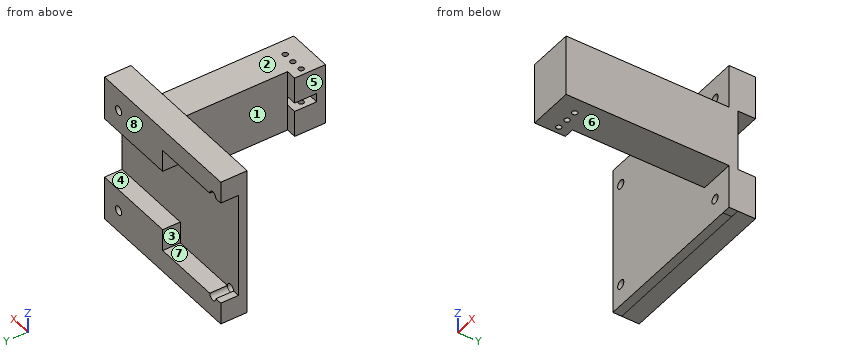
```python
from build123d import *
from build123d.topology import SkipClean

# Parameters (mm, degrees)
SKETCH3_W                = 4.167944103
SKETCH3_H                = 2.5
SKETCH3_R                = 0.3
BOSS_EXTRUDE1_DEPTH      = 3
BOSS_EXTRUDE3_DEPTH      = 3
BOSS_EXTRUDE4_DEPTH      = 8
SKETCH7_R                = 0.5
CUT_EXTRUDE1_DEPTH       = 1
BOSS_EXTRUDE5_DEPTH      = 1
BOSS_EXTRUDE5_DEPTH_BACK = 1
SKETCH8_W                = 4.167944103
SKETCH8_H                = 1
SKETCH8_W_2              = 1
BOSS_EXTRUDE6_START      = -3.5
BOSS_EXTRUDE6_OUTLINE_W  = 4.167944103
BOSS_EXTRUDE6_OUTLINE_H  = 1
BOSS_EXTRUDE6_DEPTH      = 7
BOSS_EXTRUDE7_START      = -3.5
BOSS_EXTRUDE7_OUTLINE_W  = 1
BOSS_EXTRUDE7_OUTLINE_H  = 18.5
BOSS_EXTRUDE7_DEPTH      = 7
BOSS_EXTRUDE8_START      = 2
SKETCH9_R                = 0.5
BOSS_EXTRUDE8_DEPTH      = 2
BOSS_EXTRUDE9_DEPTH      = 8.5
BOSS_EXTRUDE9_DEPTH_BACK = 8.5
SKETCH8_7_W              = 1
SKETCH8_7_H              = 1


# Read off the part's stored shape, not the designer's step: Boss-Extrude6, Boss-Extrude7
with BuildPart() as part:
    # Sketch3 → Boss-Extrude1 (new body)
    with BuildSketch(Plane.XY):
        with Locations((0.002500359, -0.178234892)):
            Rectangle(SKETCH3_W, SKETCH3_H)
        with Locations((-1.297499642, -0.208485146)):
            Circle(SKETCH3_R, mode=Mode.SUBTRACT)
        with Locations((0.002500358, -0.178234892)):
            Circle(SKETCH3_R, mode=Mode.SUBTRACT)
        with Locations((1.302500358, -0.208485146)):
            Circle(SKETCH3_R, mode=Mode.SUBTRACT)
    extrude(amount=BOSS_EXTRUDE1_DEPTH)

    # Sketch6 → Boss-Extrude3 (add)
    with BuildSketch(Plane.XY):
        Polygon((-0.91352759, 1.071765108), (2.08647241, 1.071765108), (2.08647241, 17.071765108), (-15.91352759, 17.071765108), (-15.91352759, 16.071765108), (-0.91352759, 16.071765108), align=None)
    extrude(amount=BOSS_EXTRUDE3_DEPTH)

    # Sketch6_5 → Boss-Extrude4 (add)
    with BuildSketch(Plane.XY):
        Polygon((-0.91352759, 16.071765108), (2.08647241, 16.071765108), (2.08647241, 17.071765108), (-15.91352759, 17.071765108), (-15.91352759, 16.071765108), align=None)
    extrude(amount=BOSS_EXTRUDE4_DEPTH)


with BuildPart() as body_2:
    # Mirror4: mirrored copy
    add(part.part.mirror(Plane(origin=(0, 0, -0.5), x_dir=(1, 0, 0), z_dir=(0, 0, -1))))


with BuildPart() as cut_extrude1_tool:
    # Sketch7 → Cut-Extrude1 (new body)
    with BuildSketch(Plane(origin=(0, 17.071765108, 0), x_dir=(1, 0, 0), z_dir=(0, 1, 0))):
        with Locations(Location((-14.61352759, -5.5, 0), (0, 0, 270))):
            Circle(SKETCH7_R)
        with Locations(Location((-14.61352759, 6.5, 0), (0, 0, 270))):
            Circle(SKETCH7_R)
        with Locations(Location((0.78647241, -5.5, 0), (0, 0, 270))):
            Circle(SKETCH7_R)
        with Locations(Location((0.78647241, 6.5, 0), (0, 0, 270))):
            Circle(SKETCH7_R)
    extrude(amount=-CUT_EXTRUDE1_DEPTH)


with BuildPart() as part_1:
    add(part.part)

    # Cut-Extrude1: cut by cut_extrude1_tool
    add(cut_extrude1_tool.part, mode=Mode.SUBTRACT)



with BuildPart() as body_2_1:
    add(body_2.part)

    # Cut-Extrude1: cut by cut_extrude1_tool
    add(cut_extrude1_tool.part, mode=Mode.SUBTRACT)


with BuildPart() as part_2:
    add(part_1.part)

    add(body_2_1.part)  # Boss-Extrude5 merges body 2
    # Sketch8 → Boss-Extrude5 (add, two sides: drawn at the far end of the back side and taken through both)
    with BuildSketch(Plane(origin=(0, 0, -0.5), x_dir=(-1, 0, 0), z_dir=(0, 0, -1)).offset(-BOSS_EXTRUDE5_DEPTH_BACK)):
        Polygon((-2.08647241, 16.071765108), (-2.08647241, 1.071765108), (0.91352759, 1.071765108), (0.91352759, 16.071765108), (15.91352759, 16.071765108), (15.91352759, 17.071765108), (-2.08647241, 17.071765108), align=None)
        Polygon((-2.08647241, 17.071765108), (-2.08647241, -1.428234892), (-2.08647241, -2.428234892), (-3.08647241, -2.428234892), (-3.08647241, 17.071765108), align=None)
        with Locations((-0.002500359, -1.928234892)):
            Rectangle(SKETCH8_W, SKETCH8_H)
        with Locations((-2.58647241, 16.571765108)):
            Rectangle(SKETCH8_W_2, SKETCH8_H)
    extrude(amount=BOSS_EXTRUDE5_DEPTH + BOSS_EXTRUDE5_DEPTH_BACK)

    # Boss-Extrude6 outline → Boss-Extrude6 (add)
    with BuildSketch(Plane(origin=(0, 0, -0.5), x_dir=(-1, 0, 0), z_dir=(0, 0, -1)).offset(BOSS_EXTRUDE6_START)):
        with Locations((-0.002500359, -1.928234892)):
            Rectangle(BOSS_EXTRUDE6_OUTLINE_W, BOSS_EXTRUDE6_OUTLINE_H)
    extrude(amount=BOSS_EXTRUDE6_DEPTH)

    # Boss-Extrude7 outline → Boss-Extrude7 (add)
    with BuildSketch(Plane(origin=(0, 0, -0.5), x_dir=(-1, 0, 0), z_dir=(0, 0, -1)).offset(BOSS_EXTRUDE7_START)):
        with Locations((-2.58647241, 6.821765108)):
            Rectangle(BOSS_EXTRUDE7_OUTLINE_W, BOSS_EXTRUDE7_OUTLINE_H)
    extrude(amount=BOSS_EXTRUDE7_DEPTH)

    # Sketch9 → Boss-Extrude8 (add)
    # profile 1 of 2: a face of its own
    with SkipClean():  # the faces are left unmerged after this step: merging them gives an invalid solid
        with BuildSketch(Plane(origin=(0, 17.071765108, 0), x_dir=(1, 0, 0), z_dir=(0, 1, 0)).offset(BOSS_EXTRUDE8_START)):
            with BuildLine():
                Line((-6.41352759, 6.5), (-6.41352759, 4))
                Line((-6.41352759, 4), (3.08647241, 4))
                Line((3.08647241, 4), (3.08647241, 9))
                Line((3.08647241, 9), (-15.91352759, 9))
                Line((-15.91352759, 9), (-15.91352759, 6.5))
                Line((-15.91352759, 6.5), (-15.11352759, 6.5))
                ThreePointArc((-15.11352759, 6.5), (-14.61352759, 7), (-14.11352759, 6.5))
                Line((-14.11352759, 6.5), (-6.41352759, 6.5))
            make_face()
            with Locations((0.78647241, 6.5)):
                Circle(SKETCH9_R, mode=Mode.SUBTRACT)
        # profile 2 of 2: a face of its own
        with BuildSketch(Plane(origin=(0, 17.071765108, 0), x_dir=(1, 0, 0), z_dir=(0, 1, 0)).offset(BOSS_EXTRUDE8_START)):
            with BuildLine():
                Line((-15.91352759, -5.5), (-15.91352759, -8))
                Line((-15.91352759, -8), (3.08647241, -8))
                Line((3.08647241, -8), (3.08647241, -5.5))
                Line((3.08647241, -5.5), (3.08647241, -3))
                Line((3.08647241, -3), (-6.41352759, -3))
                Line((-6.41352759, -3), (-6.41352759, -5.5))
                Line((-6.41352759, -5.5), (-14.11352759, -5.5))
                ThreePointArc((-14.11352759, -5.5), (-14.61352759, -6), (-15.11352759, -5.5))
                Line((-15.11352759, -5.5), (-15.91352759, -5.5))
            make_face()
            with Locations((0.78647241, -5.5)):
                Circle(SKETCH9_R, mode=Mode.SUBTRACT)
        extrude(amount=-BOSS_EXTRUDE8_DEPTH)

    # Sketch8_7 → Boss-Extrude9 (add, two sides: drawn at the far end of the back side and taken through both)
    with SkipClean():  # the faces are left unmerged after this step: merging them gives an invalid solid
        with BuildSketch(Plane(origin=(0, 0, -0.5), x_dir=(-1, 0, 0), z_dir=(0, 0, -1)).offset(-BOSS_EXTRUDE9_DEPTH_BACK)):
            with Locations((-2.58647241, 16.571765108)):
                Rectangle(SKETCH8_7_W, SKETCH8_7_H)
        extrude(amount=BOSS_EXTRUDE9_DEPTH + BOSS_EXTRUDE9_DEPTH_BACK)


solid = part_2.part
```
Source: CAD feature listing. Evaluate the final solid. Frame: model axes, mm. Face numbers are marked on the shaded views. A direction names the side the tool comes from. Round coordinates to 2 decimals unless told otherwise and drop trailing zeros. Loops run counter-clockwise (first coordinate to the right, second up) from the corner with the lowest first, then second, coordinate; pieces in that order, holes last.
1. Section query B-B on z = -1.75. Output: boundary loops of the cut face in (x, y).
2. Access query for the marked faces 1, 2, 3, 4 and 5. Directions: +Z, -Z, +X, -X, +Y, -Y. A direction counts if a zero-diameter tool reaches every point of the face in a straight line with its end or side. Return the directions, or none.
3. Contact query for flat-ended pins moving along their axis: pin 1 (1 mm diameter, centred on y = 9.5, z = -4, fed in from -X); pin 2 (1.5 mm diameter, centred on x = 0.5, y = 13, fed in from +Z); pin 3 (10 mm diameter, centred on x = -13, z = 6, fed in from -Y); pin 4 (3 mm diameter, centred on y = 2, z = -7, fed in from +X). Output: stop coordinate, or through.
4. Ray query, L1, parallel to Y at x = 0, z = 0.75; L2, parallel to Y at x = -4, z = 5.5; L3, parallel to Y at x = -7, z = 0. Return the intervals inside material, ascending.
5. Section query A-A on x = -5. Output: boundary loops of the cut face in (y, z).
6. Section query D-D on x = -7.75. Output: boundary loops of the cut face in (y, z).
7. Section query C-C on z = 3.75. Output: boundary loops of the cut face in (x, y), and give its area (3 significant figures).
8. Mould query, pull axis Z, two halves, no side actions, for the marked faces 6, 7 and 8. Classes: released by +Z, released by -Z, zero draft, split by the parting line, or undercut.
Answers below:
1. outline: (-15.91, 16.07) - (-0.91, 16.07) - (-0.91, 1.07) - (-2.08, 1.07) - (-2.08, -2.43) - (3.09, -2.43) - (3.09, 17.07) - (-15.91, 17.07) - close; hole circle Ø0.6 at (-1.3, -0.21); hole circle Ø0.6 at (0, -0.18); hole circle Ø0.6 at (1.3, -0.21)
2. face 1: +Z, -Z, -X
2. face 2: +Z, +X, -X, -Y
2. face 3: -X, +Y
2. face 4: +X, -X, +Y
2. face 5: +Z, -Z, -X, -Y
3. pin 1: stops at x = -0.91
3. pin 2: stops at z = 3
3. pin 3: stops at y = 16.07
3. pin 4: passes through
4. L1: y = -2.43 to -0.48, 0.12 to 17.07
4. L2: y = 16.07 to 19.07
4. L3: y = 16.07 to 17.07
5. outline: (16.07, -9) - (19.07, -9) - (19.07, -4) - (17.07, -4) - (17.07, 3) - (19.07, 3) - (19.07, 8) - (16.07, 8) - close
6. outline: (16.07, -9) - (19.07, -9) - (19.07, -6.5) - (17.07, -6.5) - (17.07, 5.5) - (19.07, 5.5) - (19.07, 8) - (16.07, 8) - close
7. outline: (-15.91, 16.07) - (3.09, 16.07) - (3.09, 19.07) - (-6.41, 19.07) - (-6.41, 17.07) - (-15.91, 17.07) - close
7. area: 38.0 mm2
8. face 6: released by -Z
8. face 7: undercut
8. face 8: zero draft
